Verification items for the finished model (mm, model axes). Round coordinates to 2 decimals unless told otherwise and drop trailing zeros. Write each loop counter-clockwise with the first axis right and the second up, starting at its lowest first coordinate (ties: lowest second). Pieces come first, ordered by that corner, then holes. Notation, with made-up numbers: M 58,51.25 L 80,51.25 A7 cw 80,57.25 Z; hole C 59,-4 d4. An arc over 180 degrees is marked long. One line per question, with ' | ' between items.
Autodesk Inventor part; units mm, degrees
ref_plane "YZ Plane" through (0, 0, 0) normal (1, 0, 0) x (0, 1, 0)
ref_plane "XZ Plane" through (0, 0, 0) normal (0, 1, 0) x (-1, 0, 0)
ref_plane "XY Plane" through (0, 0, 0) normal (0, 0, 1) x (1, 0, 0)
sketch "Sketch1" plane through (0, 0, 0) normal (0, 0, 1) x (1, 0, 0)
  circle A0 centre (0, 0) radius 19.05
  circle A1 centre (0, 0) radius 6.35
  point P0 (0, -19.05)
  point P1 (0, 19.05)
  dimension "d0" = 38.1
  dimension "d1" = 12.7
extrude "Extrusion1" add sketch "Sketch1" along normal blind 9.525
chamfer "Chamfer1" distance 2 angle 45 1 edges at (-6.35, 0, 9.525)
fillet "Fillet2" radius 3.175 1 edges at (-19.05, 0, 9.525)
properties part number "PIVOT_SPACERS,TREBUCHET" material "Wood (Oak)"
1. Section check A-A, the plane y = 0. Record the cut outline in (x, z) (3 decimals).
Results:
outline: M -19.05,0 L -6.35,0 L -6.35,7.525 L -8.35,9.525 L -15.875,9.525 A3.175 ccw -19.05,6.35 Z; M 6.35,0 L 19.05,0 L 19.05,6.35 A3.175 ccw 15.875,9.525 L 8.35,9.525 L 6.35,7.525 Z
2. Mould release check, pull along Y, two halves, no side actions. Record for faces 1 (the face through (-15.12, 11.59, 3.13)), 2 (the face through (-1.38, 6.2, 3.71)), 3 (the face through (7, -7, 9.525)): pulls with the +Y half, pulls with the -Y half, needs draft (parallel to the pull), parting line crosses it, or undercut.
Results:
face 1: parting line crosses it | face 2: undercut | face 3: needs draft
3. Section check C-C, the plane z = 3.75. Record the cut outline in (x, y).
Results:
outline: C 0,0 d38.1; hole C 0,0 d12.7
4. Go/stop test with flat-tipped pins: P1, Ø4, axis at x = -9.5, z = 6, coming from the -Y side; P2, Ø2, axis at x = -1, z = 6.5, coming from the +Y side; P3, Ø2, axis at x = 1.5, z = 8.5, coming from the -Y side. Record where each tip stops, or that it passes through.
Results:
P1: stops at y = -17.51 | P2: stops at y = 19.05 | P3: stops at y = -18.78
5. Section check D-D, the plane z = 8.5. Record the cut outline in (x, y) (3 decimals), then the cut area to 3 significant figures.
Results:
outline: C 0,0 d36.423; hole C 0,0 d14.65 | area: 873 mm2
6. Thickness scan on line 1 (Y direction, x = 0, z = 2.25); line 2 (Y direction, x = 0.5, z = 8); line 3 (X direction, y = 5.5, z = 0.75). Record the ranges inside material, lowest first.
Results:
line 1: y = -19.05 to -6.35, 6.35 to 19.05 | line 2: y = -18.58 to -6.81, 6.81 to 18.58 | line 3: x = -18.24 to -3.17, 3.17 to 18.24
